```python
from build123d import *

# Parameters (mm, degrees)
SKETCH2_W           = 80
SKETCH2_H           = 30
BOSS_EXTRUDE1_DEPTH = 15
CUT_EXTRUDE4_DEPTH  = 16
CUT_EXTRUDE5_DEPTH  = 16


with BuildPart() as part:
    # Sketch2 → Boss-Extrude1 (new body)
    with BuildSketch(Plane(origin=(0, 0, 0), x_dir=(1, 0, 0), z_dir=(0, 1, 0))):
        Rectangle(SKETCH2_W, SKETCH2_H)
    extrude(amount=BOSS_EXTRUDE1_DEPTH)

    # Sketch4 → Cut-Extrude4 (cut, through all)
    with BuildSketch(Plane(origin=(0, 15, 0), x_dir=(1, 0, 0), z_dir=(0, 1, 0))):
        with BuildLine():
            Line((25, 15), (40, 15))
            Line((40, 15), (40, 0))
            ThreePointArc((40, 0), (35.606601718, 10.606601718), (25, 15))
        make_face()
    extrude(amount=-CUT_EXTRUDE4_DEPTH, mode=Mode.SUBTRACT)

    # Sketch5 → Cut-Extrude5 (cut, through all)
    with BuildSketch(Plane(origin=(0, 15, 0), x_dir=(1, 0, 0), z_dir=(0, 1, 0))):
        with BuildLine():
            Line((40, 0), (40, -15))
            Line((40, -15), (25, -15))
            ThreePointArc((25, -15), (35.606601718, -10.606601718), (40, 0))
        make_face()
    extrude(amount=-CUT_EXTRUDE5_DEPTH, mode=Mode.SUBTRACT)


solid = part.part
```
Design review of the part built by this model. Coordinates are the model's own, in mm. Coordinates: 2 decimals unless noted, no trailing zeros. Loops run counter-clockwise (first coordinate to the right, second up) from the corner with the lowest first, then second, coordinate; pieces in that order, holes last.
Q1. To check wall thickness, follow line 1 (Z direction, x = 27, y = 2.5); line 2 (X direction, y = 4.5, z = 13.5); line 3 (X direction, y = 2.5, z = -4). State the ranges of each line that lie inside material, in increasing order.
Reported:
line 1: z = -14.87 to 14.87
line 2: x = -40 to 31.54
line 3: x = -40 to 39.46
Q2. For pin 1 (2 mm diameter, centred on x = 28, y = 7.5, fed in from +Z); pin 2 (1.5 mm diameter, centred on x = 30.5, y = 2.5, fed in from +Z); pin 3 (1.5 mm diameter, centred on y = 11.5, z = -1, fed in from +X), all flat-tipped, find the tip position at first contact; note any pin that passes through.
Reported:
pin 1: stops at z = 14.87
pin 2: stops at z = 14.23
pin 3: stops at x = 40
Q3. We need section B-B on z = 8.75. State the section outline as (x, y) points.
Reported:
outline: (-40, 0) - (37.18, 0) - (37.18, 15) - (-40, 15) - close
Q4. We need section A-A on y = 1.75. State the section outline as (x, z) points, and give its area (3 significant figures).
Reported:
outline: (-40, -15) - (25, -15) arc R15 ccw to (25, 15) - (-40, 15) - close
area: 2,300 mm2
Q5. We need section C-C on x = 35. State the section outline as (y, z) points, and give its area (3 significant figures).
Reported:
outline: (0, -11.18) - (15, -11.18) - (15, 11.18) - (0, 11.18) - close
area: 335 mm2
